Part model, mm, in its own coordinate system. A direction names the side the tool comes from. Round coordinates to 2 decimals unless told otherwise and drop trailing zeros. Write each loop counter-clockwise with the first axis right and the second up, starting at its lowest first coordinate (ties: lowest second). Pieces come first, ordered by that corner, then holes. Notation, with made-up numbers: M 81,4.25 L 103,4.25 A21 cw 103,38.25 Z; hole C 39,50 d10. An arc over 180 degrees is marked long. Use one line per item in the form item = value. Start each with the question number.
Item 1: Probe L1, parallel to Z at x = -15, y = -2; L2, parallel to Y at x = 27.9, z = 15; L3, parallel to X at y = -1.15, z = 15.5. List the from-to ranges inside material, lowest first.
Item 2: Mould opens along Z. For faces 6 (the face through (0, -3, 0)), 7 (the face through (28, -6, 14)), 8 (the face through (27.472, -23.719, 27.594)), 9 (the face through (28, -21, 15)) say: +Z half, -Z half, draft (parallel to the pull), parting line (faces both ways), or undercut.
Item 3: Cut at D-D, the plane z = 18.75. Give the cut face in (x, y).
Item 4: Cut at A-A, the plane y = -13. Give the cut face in (x, z), then the cut area to 3 significant figures.
Item 5: Cut at B-B, the plane x = -15. Give the cut face in (y, z).
Item 6: Cut at C-C, the plane y = -6. Give the cut face in (x, z).
Item 7: Which spindle directions (+Z, -Z, +X, -X, +Y, -Y) get a long thin tool onto all of the face, cutting with end or side? Do faces 1 (the face through (-25.5, -15, 15)), 2 (the face through (28, -14, 22)), 3 (the face through (27.472, -23.719, 2.406)), 4 (the face through (-27.528, -23.719, 27.594)), 5 (the face through (-27.528, -13.632, 16.524)). Say none if no direction does.
Item 8: Flat gauge pins, fed straight in: pin 1 Ø9 at (x, z) = (3.5, 11) entering from -Y; pin 2 Ø1.2 at (y, z) = (-6, 15) entering from +X. Where does each tip first touch, or does it go through?
from build123d import *

# Parameters (mm, degrees)
EXTRUDE_1_DEPTH     = 30
FILLET_1_R          = 8
SKETCH_4_R          = 1.65
CUT_EXTRUDE_1_DEPTH = 10
SKETCH_5_R          = 1.65
CUT_EXTRUDE_2_DEPTH = 10
SKETCH_6_R          = 1
CUT_EXTRUDE_3_DEPTH = 10
SKETCH_7_R          = 1.5
CUT_EXTRUDE_4_DEPTH = 10


with BuildPart() as part:
    # 草图1 → 凸台-拉伸1 (new body)
    with BuildSketch(Plane.XY):
        Polygon((0, 0), (29.5, 0), (29.5, -26), (25.5, -26), (25.5, -4), (0, -4), (-25.5, -4), (-25.5, -26), (-29.5, -26), (-29.5, 0), align=None)
    extrude(amount=EXTRUDE_1_DEPTH)

    # 圆角1
    fillet_1_edges = [part.edges().sort_by_distance(p)[0] for p in [
        (27.5, -26, 0),
        (-27.5, -26, 0),
        (-27.5, -26, 30),
        (27.5, -26, 30),
    ]]
    fillet(fillet_1_edges, radius=FILLET_1_R)

    # 草图4 → 切除-拉伸1 (cut)
    with BuildSketch(Plane(origin=(0, 0, 0), x_dir=(1, 0, 0), z_dir=(0, 1, 0))):
        with Locations((15, -7.5)):
            Circle(SKETCH_4_R)
        with Locations((-15, -7.5)):
            Circle(SKETCH_4_R)
        with Locations((-15, -15.5)):
            Circle(SKETCH_4_R)
        with Locations((15, -15.5)):
            Circle(SKETCH_4_R)
    extrude(amount=-CUT_EXTRUDE_1_DEPTH, mode=Mode.SUBTRACT)

    # 草图5 → 切除-拉伸2 (cut)
    with BuildSketch(Plane.ZY.offset(29.5)):
        with Locations((15, -13)):
            Circle(SKETCH_5_R)
    extrude(amount=-CUT_EXTRUDE_2_DEPTH, mode=Mode.SUBTRACT)

    # 草图6 → 切除-拉伸3 (cut)
    with BuildSketch(Plane(origin=(29.5, 0, 0), x_dir=(0, 0, -1), z_dir=(1, 0, 0))):
        with Locations((-15, -6)):
            Circle(SKETCH_6_R)
        with Locations((-8, -13)):
            Circle(SKETCH_6_R)
        with Locations((-15, -20)):
            Circle(SKETCH_6_R)
        with Locations((-22, -13)):
            Circle(SKETCH_6_R)
    extrude(amount=-CUT_EXTRUDE_3_DEPTH, mode=Mode.SUBTRACT)

    # 草图7 → 切除-拉伸4 (cut)
    with BuildSketch(Plane(origin=(29.5, 0, 0), x_dir=(0, 0, -1), z_dir=(1, 0, 0))):
        with Locations((-15, -13)):
            Circle(SKETCH_7_R)
    extrude(amount=-CUT_EXTRUDE_4_DEPTH, mode=Mode.SUBTRACT)


solid = part.part
Model answer:
q1.L1 = 0 to 5.85, 9.15 to 13.85, 17.15 to 30
q1.L2 = -26 to -21, -19 to -14.5, -11.5 to -7, -5 to 0
q1.L3 = -29.5 to -16.65, -13.35 to 13.35, 16.65 to 29.5
q2.face_6 = -Z half
q2.face_7 = undercut
q2.face_8 = +Z half
q2.face_9 = undercut
q3.outline = M -29.5,-26 L -25.5,-26 L -25.5,-4 L 25.5,-4 L 25.5,-26 L 29.5,-26 L 29.5,0 L -29.5,0 Z
q4.outline = M -29.5,0 L -25.5,0 L -25.5,13.35 L -29.5,13.35 Z; M -29.5,16.65 L -25.5,16.65 L -25.5,30 L -29.5,30 Z; M 25.5,0 L 29.5,0 L 29.5,7 L 25.5,7 Z; M 25.5,9 L 29.5,9 L 29.5,13.5 L 25.5,13.5 Z; M 25.5,16.5 L 29.5,16.5 L 29.5,21 L 25.5,21 Z; M 25.5,23 L 29.5,23 L 29.5,30 L 25.5,30 Z
q4.area = 199 mm²
q5.outline = M -4,0 L 0,0 L 0,5.85 L -4,5.85 Z; M -4,9.15 L 0,9.15 L 0,13.85 L -4,13.85 Z; M -4,17.15 L 0,17.15 L 0,30 L -4,30 Z
q6.outline = M -29.5,0 L -25.5,0 L -25.5,30 L -29.5,30 Z; M 25.5,0 L 29.5,0 L 29.5,14 L 25.5,14 Z; M 25.5,16 L 29.5,16 L 29.5,30 L 25.5,30 Z
q7.face_1 = +Z, -Z, -Y
q7.face_2 = +X
q7.face_3 = -Z, +X, -X, -Y
q7.face_4 = +Z, +X, -X, -Y
q7.face_5 = -X
q8.pin_1 = -4
q8.pin_2 = -25.5
